Source: three-view drawing plus pictorial views. Frame: mm from the lowest corner of the part. A direction names the side the tool comes from. Give positions to 0.01 mm unless a question says otherwise; leave off trailing zeros. Answer as a JSON object with one key per item and string values. Group by question number.
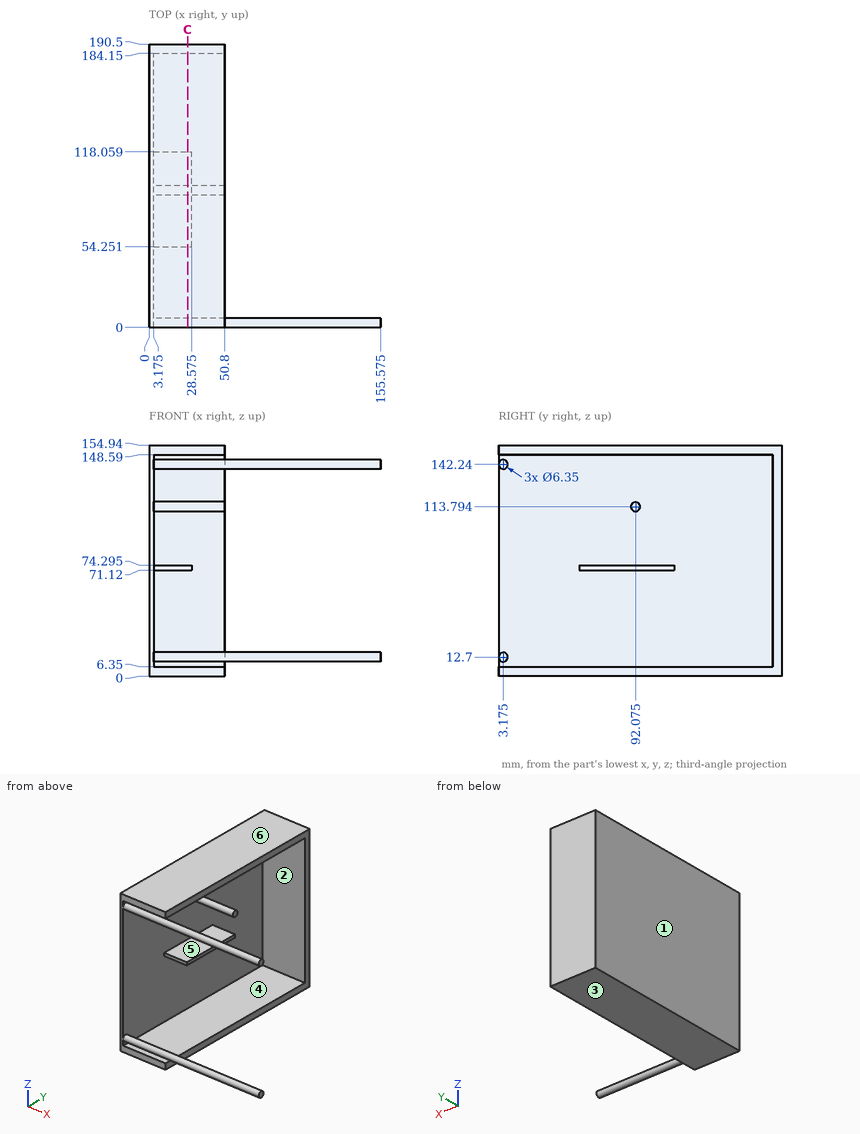
(1) Material intervals for line 1 (Z direction, x = 32, y = 137); line 2 (Y direction, x = 28, z = 106); line 3 (X direction, y = 51, z = 104) (1 decimal), sorted ascending. Write a range as from..to.
(2) Mould query, pull axis Z, two halves, no side actions, for the marked faces 3, 4, 5 and 6. Classes: pulls with the +Z half, pulls with the -Z half, needs draft (parallel to the pull), parting line crosses it, or undercut.
(3) Section query C-C on x = 26. State how many separate pieces and enclosed holes the cut face has, plus the area to 3 significant figures.
(4) Access query for the marked faces 1 and 2. Directions: +Z, -Z, +X, -X, +Y, -Y. A direction counts if a zero-diameter tool reaches every point of the face in a straight line with its end or side. Return the directions, or none.
(5) First-contact query: pin 1 (4 mm diameter, centred on x = 54.5, y = 43, fed in from +Z) (1 decimal); pin 2 (1.6 mm diameter, centred on y = 75, z = 73, fed in from +X) (3 decimals); pin 3 (7 mm diameter, centred on y = 92, z = 115, fed in from +X); pin 4 (2 mm diameter, centred on y = 90, z = 32, fed in from +X) (3 decimals). Flat tips, straight axial feed; report the tip coordinate or a pass-through.
Result:
{
 "1": {"line 1": "0..6.35, 148.59..154.94", "line 2": "184.15..190.5", "line 3": "0..3.2"},
 "2": {"face 3": "pulls with the -Z half", "face 4": "undercut", "face 5": "undercut", "face 6": "pulls with the +Z half"},
 "3": {"separate pieces": "5", "enclosed holes": "0", "area": "3,620 mm²"},
 "4": {"face 1": "+Z, -Z, -X, +Y, -Y", "face 2": "+X"},
 "5": {"pin 1": "through", "pin 2": "x = 28.575", "pin 3": "x = 50.8", "pin 4": "x = 3.175"}
}
